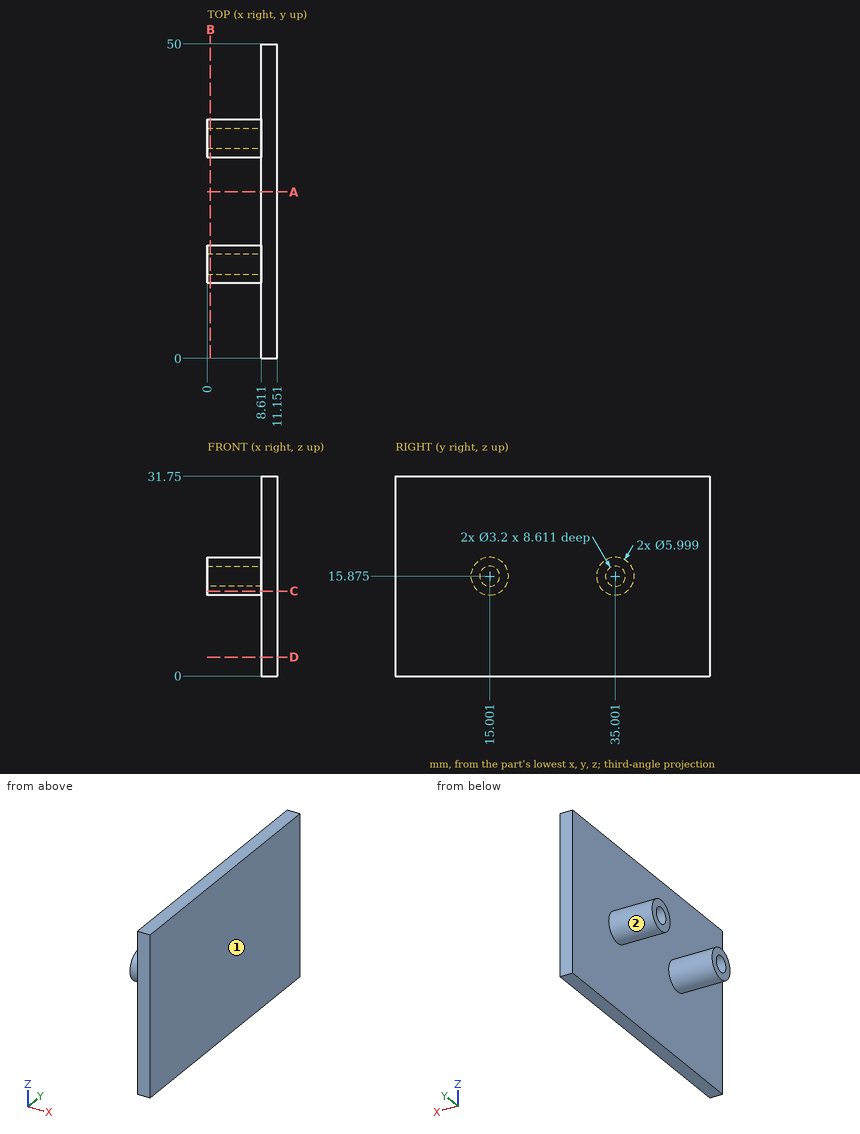
Verification items for this drawing (mm, ordinates from the low corner). Round coordinates to 2 decimals unless told otherwise and drop trailing zeros. Write each loop counter-clockwise with the first axis right and the second up, starting at its lowest first coordinate (ties: lowest second). Pieces come first, ordered by that corner, then holes. Notation, with made-up numbers: (74.5, 72.5) - (104.5, 72.5) arc R24 ccw to (104.5, 109.5) - close; hole circle Ø4 at (46.5, 1.25). An arc over 180 degrees is marked (long way). Answer as a JSON object with one key per item and string values. Group by question number.
Q1. Section check A-A, the plane y = 26.5. Enter the section's corners in (x, z).
Q2. Section check D-D, the plane z = 3. Enter the section's corners in (x, y).
Q3. Section check B-B, the plane x = 0.5. Enter the section's corners in (y, z) (1 decimal).
Q4. Section check C-C, the plane z = 13.5. Enter the section's corners in (x, y), plus the area to 3 significant figures.
Q5. Thickness scan on line 1 (X direction, y = 37.5, z = 18); line 2 (Z direction, x = 1.25, y = 35.5) (1 decimal); line 3 (Z direction, x = 1.25, y = 12.5). Record the ranges inside material, lowest first.
Q6. Mould release check, pull along Y, two halves, no side actions. Record for the marked faces 1 and 2: released by +Y, released by -Y, zero draft, split by the parting line, or undercut.
Q7. Go/stop test with flat-tipped pins: pin 1 Ø6 at (x, z) = (4, 15.5) entering from -Y; pin 2 Ø5 at (x, y) = (2, 16.5) entering from -Z (1 decimal); pin 3 Ø1.5 at (x, y) = (3.5, 30) entering from +Z; pin 4 Ø16 at (y, z) = (24, 23.5) entering from -X. Record where each tip stops, or that it passes through.
Found:
{
 "1": {"outline": "(8.61, 0) - (11.15, 0) - (11.15, 31.75) - (8.61, 31.75) - close"},
 "2": {"outline": "(8.61, 0) - (11.15, 0) - (11.15, 50) - (8.61, 50) - close"},
 "3": {"outline": "circle Ø6 at (15, 15.9); circle Ø6 at (35, 15.9); hole circle Ø3.2 at (15, 15.9); hole circle Ø3.2 at (35, 15.9)"},
 "4": {"outline": "(0, 13.17) - (8.61, 13.17) - (8.61, 0) - (11.15, 0) - (11.15, 50) - (8.61, 50) - (8.61, 36.83) - (0, 36.83) - (0, 33.17) - (8.61, 33.17) - (8.61, 16.83) - (0, 16.83) - close", "area": "190 mm^2"},
 "5": {"line 1": "x = 8.61 to 11.15", "line 2": "z = 12.9 to 14.4, 17.4 to 18.8", "line 3": "z = 14.22 to 17.53"},
 "6": {"face 1": "zero draft", "face 2": "undercut"},
 "7": {"pin 1": "stops at y = 12", "pin 2": "stops at z = 12.9", "pin 3": "passes through", "pin 4": "stops at x = 8.61"}
}
